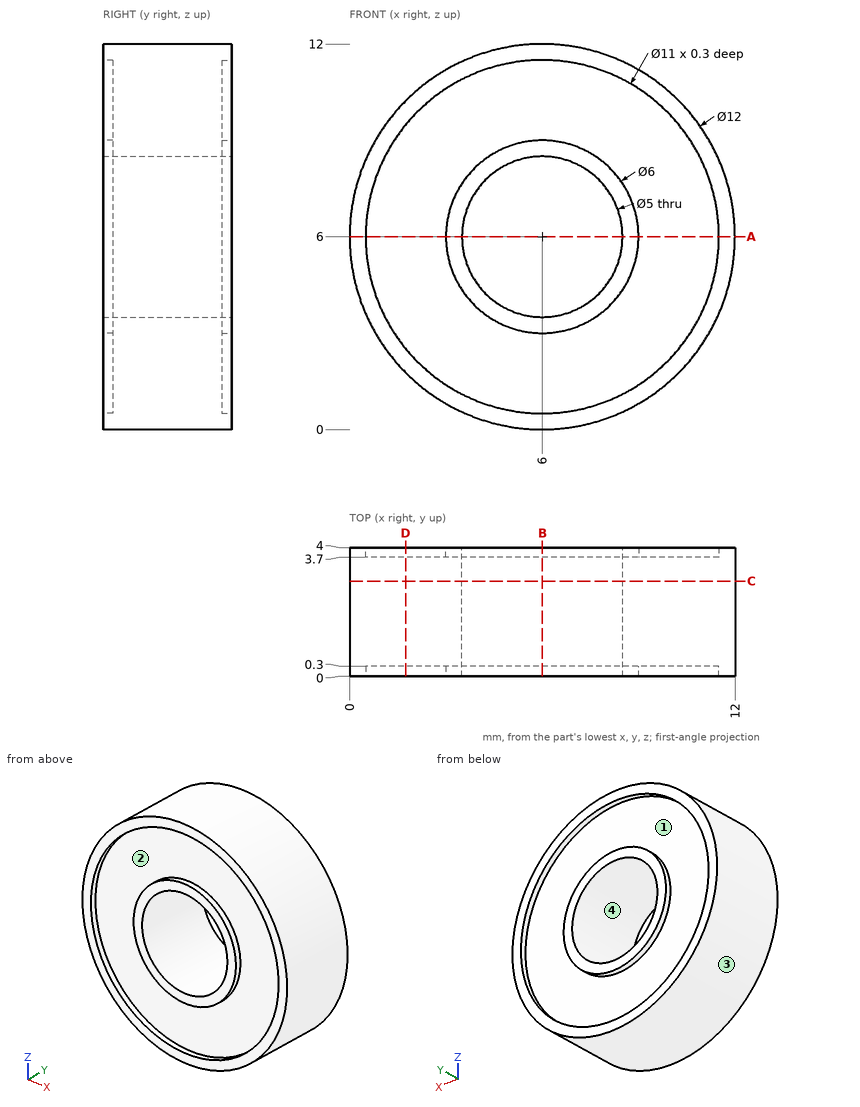
Can you work these out from the drawing? Everything is in mm from the part's minimum corner. A direction names the side the tool comes from. Give positions to 0.01 mm unless a question says otherwise; leave off trailing zeros. Order: outer loops, then holes, each group sorted by start corner. A loop starts at its lowest first (then second) coordinate and runs counter-clockwise, first axis right, second up.
1. Will these pins go through, and if not, where does the flat tip stop? P1, Ø2, axis at y = 2.5, z = 3.5, coming from the -X side; P2, Ø1.5, axis at x = 5, z = 2, coming from the -Y side; P3, Ø1.5, axis at y = 3.5, z = 4.5, coming from the -X side.
2. Suppose I cut it at A-A (z = 6). List the corners of the cut face in (x, y) for me, plus the area to 3 significant figures.
3. Suppose I cut it at D-D (x = 1.75). List the corners of the cut face in (y, z) for me.
4. Suppose I cut it at B-B (x = 6). List the corners of the cut face in (y, z) for me.
5. For the marked faces 1 and 2, which set-ups out of +Z, -Z, +X, -X, +Y, -Y let a thin tool reach every point of the face, with its end or its side?
6. I need wall thicknesses on L1, parallel to Z at x = 6, y = 0.25; L2, parallel to Z at x = 6, y = 1.9; L3, parallel to X at y = 1.6, z = 7.5. Which ranges of each line are inside material? Lowest first, please.
7. We'd pull the mould along X, two halves only. Please class the marked faces 3 and 4: pulls with the +X half, pulls with the -X half, needs draft (parallel to the pull), parting line crosses it, or undercut.
8. Suppose I cut it at C-C (y = 2.95). List the corners of the cut face in (x, z) for me, plus the area to 3 significant figures.
Solved:
1. P1: stops at x = 0.19
1. P2: stops at y = 0.3
1. P3: stops at x = 0.05
2. outline: (0, 0) - (0.5, 0) - (0.5, 0.3) - (3, 0.3) - (3, 0) - (3.5, 0) - (3.5, 4) - (3, 4) - (3, 3.7) - (0.5, 3.7) - (0.5, 4) - (0, 4) - close; (8.5, 0) - (9, 0) - (9, 0.3) - (11.5, 0.3) - (11.5, 0) - (12, 0) - (12, 4) - (11.5, 4) - (11.5, 3.7) - (9, 3.7) - (9, 4) - (8.5, 4) - close
2. area: 25.0 mm2
3. outline: (0, 1.76) - (4, 1.76) - (4, 2.51) - (3.7, 2.51) - (3.7, 9.49) - (4, 9.49) - (4, 10.24) - (0, 10.24) - (0, 9.49) - (0.3, 9.49) - (0.3, 2.51) - (0, 2.51) - close
4. outline: (0, 0) - (4, 0) - (4, 0.5) - (3.7, 0.5) - (3.7, 3) - (4, 3) - (4, 3.5) - (0, 3.5) - (0, 3) - (0.3, 3) - (0.3, 0.5) - (0, 0.5) - close; (0, 8.5) - (4, 8.5) - (4, 9) - (3.7, 9) - (3.7, 11.5) - (4, 11.5) - (4, 12) - (0, 12) - (0, 11.5) - (0.3, 11.5) - (0.3, 9) - (0, 9) - close
5. face 1: +Y
5. face 2: -Y
6. L1: z = 0 to 0.5, 3 to 3.5, 8.5 to 9, 11.5 to 12
6. L2: z = 0 to 3.5, 8.5 to 12
6. L3: x = 0.19 to 4, 8 to 11.81
7. face 3: parting line crosses it
7. face 4: undercut
8. outline: circle Ø12 at (6, 6); hole circle Ø5 at (6, 6)
8. area: 93.5 mm2
